Model file for the job. Use its own axes, mm. A direction names the side the tool comes from. Coordinates: 2 decimals unless noted, no trailing zeros. Write each loop counter-clockwise with the first axis right and the second up, starting at its lowest first coordinate (ties: lowest second). Pieces come first, ordered by that corner, then holes.
Q1. Band-saw the part on A-A, the plane z = 1.5. Write the cut outline in (x, y).
Q2. Which spindle directions (+Z, -Z, +X, -X, +Y, -Y) get a long thin tool onto all of the face, cutting with end or side? Do faces 4 (the flat face through (-3, 4, -9.625)), 5 (the flat face through (-7, 6, -11)). Say none if no direction does.
Q3. Band-saw the part on C-C, the plane x = 2. Write the cut outline in (y, z).
Q4. Drill centre lines: probe 1 along Y at (x, z) = (10, -10); probe 2 along X at (y, z) = (4.25, 5.5); probe 3 along X at (y, z) = (1.5, 6). Where is each one in solid material? Low to high.
Q5. Pull direction Z, two halves, no side cores. Call faces 1 (the cylindrical face through (16.564, 1.479, 0.1)), 2 (the flat face through (-0.035, 4.521, -10.833)), 3 (the flat face through (9, 3, 0)): released by +Z, released by -Z, zero draft, split by the parting line, or undercut.
Q6. Band-saw the part on B-B, the plane y = 2.5. Write the cut outline in (x, z), plus the area to 3 significant figures.
Q7. Band-saw the part on D-D, the plane y = 4.25. Write the cut outline in (x, z), plus the area to 3 significant figures.
Q8. Pin check, flat tips, straight feed: P1, Ø1.5, axis at x = 5, z = 9.5, coming from the +Y side; P2, Ø2.5, axis at x = -9.08, z = -5.63, coming from the +Y side. Stop position of each tip, or through.
from build123d import *

# Parameters (mm, degrees)
CROQUIS1_R              = 3.999426158
CROQUIS1_R_2            = 1.000000121
CROQUIS1_R_3            = 1.000000477
SALIENTE_EXTRUIR1_DEPTH = 3
SALIENTE_EXTRUIR2_DEPTH = 24.89496
CROQUIS3_W              = 13.299999714
CROQUIS3_H              = 2.45
SALIENTE_EXTRUIR3_DEPTH = 3
CORTAR_EXTRUIR1_DEPTH   = 24.89496
CROQUIS5_R              = 1.000000121
CROQUIS5_R_2            = 1.000000477
CORTAR_EXTRUIR2_DEPTH   = 11


with BuildPart() as part:
    # Croquis1 → Saliente-Extruir1 (new body)
    with BuildSketch(Plane(origin=(0, 0, 0), x_dir=(1, 0, 0), z_dir=(0, 1, 0))):
        with BuildLine():
            Line((4.218422555, -12.81969876), (-15.081577159, -12.81969876))
            Line((-15.081577159, -12.81969876), (-15.081577159, 12.075260967))
            Line((-15.081577159, 12.075260967), (4.218422555, 12.075260967))
            ThreePointArc((4.218422555, 12.075260967), (16.567050884, -0.372218896), (4.218422555, -12.81969876))
        make_face()
        with Locations((4.119175364, -0.372218896)):
            Circle(CROQUIS1_R, mode=Mode.SUBTRACT)
        with Locations((-9.081577367, 5.628403394)):
            Circle(CROQUIS1_R_2, mode=Mode.SUBTRACT)
        with Locations((-9.081576585, -6.371596672)):
            Circle(CROQUIS1_R_3, mode=Mode.SUBTRACT)
    extrude(amount=SALIENTE_EXTRUIR1_DEPTH)

    # Croquis2 → Saliente-Extruir2 (add)
    with BuildSketch(Plane.XY.offset(12.81969876)):
        with BuildLine():
            Line((-14.277729582, 3), (-3.885424736, 3))
            ThreePointArc((-3.885424736, 3), (-9.081577159, 6), (-14.277729582, 3))
        make_face()
    extrude(amount=-SALIENTE_EXTRUIR2_DEPTH)

    # Croquis3 → Saliente-Extruir3 (add)
    with BuildSketch(Plane(origin=(0, 3, 0), x_dir=(1, 0, 0), z_dir=(0, 1, 0))):
        with Locations((-2.431577302, -11.59469876)):
            Rectangle(CROQUIS3_W, CROQUIS3_H)
        with Locations((-2.431577302, 10.850260967)):
            Rectangle(CROQUIS3_W, CROQUIS3_H)
    extrude(amount=SALIENTE_EXTRUIR3_DEPTH)

    # Croquis4 → Cortar-Extruir1 (cut)
    with BuildSketch(Plane.XY.offset(12.81969876)):
        Polygon((-4.171577445, 6), (4.218422555, 3), (4.218422555, 6), align=None)
        with BuildLine():
            Line((-15.081577159, 0), (-16.256016644, 0))
            ThreePointArc((-16.256016644, 0), (-14.36312843, 4.855697487), (-9.683294652, 7.149162047))
            Line((-9.683294652, 7.149162047), (-9.683294652, 5.969751759))
            ThreePointArc((-9.683294652, 5.969751759), (-13.53187518, 4.024282237), (-15.081577159, 0))
        make_face()
    extrude(amount=-CORTAR_EXTRUIR1_DEPTH, mode=Mode.SUBTRACT)

    # Croquis5 → Cortar-Extruir2 (cut)
    with BuildSketch(Plane.XZ):
        with Locations((-9.081577367, -5.628403394)):
            Circle(CROQUIS5_R)
        with Locations((-9.081576585, 6.371596672)):
            Circle(CROQUIS5_R_2)
    extrude(amount=-CORTAR_EXTRUIR2_DEPTH, mode=Mode.SUBTRACT)


solid = part.part
Answer sheet:
1. outline: (-15.08, 0) - (0.28, 0) - (0.28, 3) - (-3.89, 3) arc R6 ccw to start; (7.96, 0) - (16.52, 0) - (16.52, 3) - (7.96, 3) - close
2. face 4: +X, +Y
2. face 5: +Z, -Z, +X, -X, +Y
3. outline: (0, -12.08) - (3.79, -12.08) - (3.79, -9.63) - (3, -9.63) - (3, -3.02) - (0, -3.02) - close; (0, 3.76) - (3, 3.76) - (3, 10.37) - (3.79, 10.37) - (3.79, 12.82) - (0, 12.82) - close
4. probe 1: y = 0 to 3
4. probe 2: x = -13.32 to -9.57, -8.59 to -4.85
4. probe 3: x = -14.89 to -10.01, -8.15 to 15.22
5. face 1: split by the parting line
5. face 2: zero draft
5. face 3: undercut
6. outline: (-14.54, -12.08) - (4.22, -12.08) arc R12.45 ccw to (4.22, 12.82) - (-14.54, 12.82) - close; hole circle Ø2 at (-9.08, -5.63); hole circle Ø2 at (-9.08, 6.37); hole circle Ø8 at (4.12, 0.37)
6. area: 651 mm2
7. outline: (-13.32, -12.08) - (0.72, -12.08) - (0.72, -9.63) - (-4.85, -9.63) - (-4.85, 10.37) - (0.72, 10.37) - (0.72, 12.82) - (-13.32, 12.82) - close; hole circle Ø2 at (-9.08, -5.63); hole circle Ø2 at (-9.08, 6.37)
7. area: 232 mm2
8. P1: stops at y = 3
8. P2: stops at y = 6
